```python
from build123d import *

# Parameters (mm, degrees)
F0_W         = 2.23
F0_H         = 8.65
F1_DEPTH     = 1.5
F2_DEPTH     = 31
F5_DEPTH     = 2
F6_R         = 1.5
F7_DEPTH     = 6
F8_R         = 2
F9_DEPTH     = 2.5
F10_T1_DEPTH = 13.5
F10_T3_DEPTH = 36
F10_T6_ANGLE = 90


# Not quite as in the source:
# - a fillet or chamfer that OpenCascade refuses, or shapes differently, is made with other operations: its cross-section is extruded or revolved along the edge and cut away or added
# - a feature names something its author has since deleted; it is built from what else it names


with BuildPart() as f1:
    # F0 (on Top) → F1 (new body)
    with BuildSketch(Plane.XY):
        with BuildLine():
            Line((-1.75, -15), (1.75, -15))
            ThreePointArc((1.75, -15), (3.517766953, -14.267766953), (4.25, -12.5))
            Line((4.25, -12.5), (4.25, -5.3126580607))
            add(Edge.make_bspline(
                [(4.25, -5.3126580607), (5.242489647, 0), (4.25, 5.3126580607)],
                knots=[4.2622339472, 4.2622339472, 4.2622339472, 5.1625440136, 5.1625440136, 5.1625440136], degree=2, weights=[1, 0.9003796574, 1]))
            Line((4.25, 5.3126580607), (4.25, 12.5))
            ThreePointArc((4.25, 12.5), (3.517766953, 14.267766953), (1.75, 15))
            Line((1.75, 15), (-1.75, 15))
            ThreePointArc((-1.75, 15), (-3.517766953, 14.267766953), (-4.25, 12.5))
            Line((-4.25, 12.5), (-4.25, -12.5))
            ThreePointArc((-4.25, -12.5), (-3.517766953, -14.267766953), (-1.75, -15))
        make_face()
        Rectangle(F0_W, F0_H, mode=Mode.SUBTRACT)
    extrude(amount=F1_DEPTH)

    # F0 (on Top) → F2 (join)
    with BuildSketch(Plane.XY):
        with BuildLine():
            ThreePointArc((5.75, 14), (5.017766953, 15.767766953), (3.25, 16.5))
            Line((3.25, 16.5), (-3.25, 16.5))
            ThreePointArc((-3.25, 16.5), (-5.017766953, 15.767766953), (-5.75, 14))
            Line((-5.75, 14), (-5.75, -14))
            ThreePointArc((-5.75, -14), (-5.017766953, -15.767766953), (-3.25, -16.5))
            Line((-3.25, -16.5), (5.75, -16.5))
            Line((5.75, -16.5), (5.75, 14))
        make_face()
        with BuildLine():
            ThreePointArc((4.25, -12.5), (3.517766953, -14.267766953), (1.75, -15))
            Line((1.75, -15), (-1.75, -15))
            ThreePointArc((-1.75, -15), (-3.517766953, -14.267766953), (-4.25, -12.5))
            Line((-4.25, -12.5), (-4.25, 12.5))
            ThreePointArc((-4.25, 12.5), (-3.517766953, 14.267766953), (-1.75, 15))
            Line((-1.75, 15), (1.75, 15))
            ThreePointArc((1.75, 15), (3.517766953, 14.267766953), (4.25, 12.5))
            Line((4.25, 12.5), (4.25, 5.3126580607))
            add(Edge.make_bspline(
                [(4.25, -5.3126580607), (5.242489647, 0), (4.25, 5.3126580607)],
                knots=[4.2622339472, 4.2622339472, 4.2622339472, 5.1625440136, 5.1625440136, 5.1625440136], degree=2, weights=[1, 0.9003796574, 1]))
            Line((4.25, -5.3126580607), (4.25, -12.5))
        make_face(mode=Mode.SUBTRACT)
    extrude(amount=F2_DEPTH)

    # F4 (on face) → F5 (cut)
    with BuildSketch(Plane.YZ.offset(5.75)):
        with BuildLine():
            ThreePointArc((6.52, 16.25), (-4.6103362133, 20.8603362133), (0, 9.73))
            ThreePointArc((0, 9.73), (4.6103362133, 11.6396637867), (6.52, 16.25))
        make_face()
    extrude(amount=-F5_DEPTH, mode=Mode.SUBTRACT)

    # F6
    f6_edges = [f1.edges().sort_by_distance(p)[0] for p in [
        (5.75, -1.25, 0),
    ]]
    fillet(f6_edges, radius=F6_R)

    # F3 (on face) → F7 (join)
    with BuildSketch(Plane.XY.offset(31)):
        with BuildLine():
            Line((2.6164813973, -14.8450394427), (2.6164813973, -16.5))
            Line((2.6164813973, -16.5), (5.75, -16.5))
            Line((5.75, -16.5), (5.75, -13.5683528888))
            Line((5.75, -13.5683528888), (4.0102261181, -13.5683528888))
            ThreePointArc((4.0102261181, -13.5683528888), (3.4386554151, -14.3434866121), (2.6164813973, -14.8450394427))
        make_face()
        with BuildLine():
            Line((4.0102261181, -13.5683528888), (5.75, -13.5683528888))
            Line((5.75, -13.5683528888), (5.75, -9.473525919))
            Line((5.75, -9.473525919), (4.25, -9.473525919))
            Line((4.25, -9.473525919), (4.25, -12.5))
            ThreePointArc((4.25, -12.5), (4.18932012, -13.0474644759), (4.0102261181, -13.5683528888))
        make_face()
        with BuildLine():
            Line((-1.75, -15), (-1.75, -16.5))
            Line((-1.75, -16.5), (2.6164813973, -16.5))
            Line((2.6164813973, -16.5), (2.6164813973, -14.8450394427))
            ThreePointArc((2.6164813973, -14.8450394427), (2.190114413, -14.9609549576), (1.75, -15))
            Line((1.75, -15), (-1.75, -15))
        make_face()
    extrude(amount=F7_DEPTH)

    # F8
    f8_edges = [f1.edges().sort_by_distance(p)[0] for p in [
        (-1.75, -15.75, 37),
        (5, -9.473526, 37),
    ]]
    fillet(f8_edges, radius=F8_R)

    # F3 (on face) → F9 (cut)
    with BuildSketch(Plane.XY.offset(31)):
        with BuildLine():
            Line((2.6164813973, -14.8450394427), (2.6164813973, -16.5))
            Line((2.6164813973, -16.5), (5.75, -16.5))
            Line((5.75, -16.5), (5.75, -13.5683528888))
            Line((5.75, -13.5683528888), (4.0102261181, -13.5683528888))
            ThreePointArc((4.0102261181, -13.5683528888), (3.4386554151, -14.3434866121), (2.6164813973, -14.8450394427))
        make_face()
    extrude(amount=F9_DEPTH, mode=Mode.SUBTRACT)

    # F10: fillet of radius 2 on 2 edges, made by hand

    # F10_s2 → F10_t1 (cut)
    with BuildSketch(Plane.XY.offset(28.5)):
        with BuildLine():
            ThreePointArc((5.75, -14.5), (5.1642135624, -15.9142135624), (3.75, -16.5))
            Line((3.75, -16.5), (5.75, -16.5))
            Line((5.75, -16.5), (5.75, -14.5))
        make_face()
    extrude(amount=F10_T1_DEPTH, mode=Mode.SUBTRACT)

    # F10_s4 → F10_t3 (cut)
    with BuildSketch(Plane.XY):
        with BuildLine():
            ThreePointArc((5.75, -14.5), (5.1642135624, -15.9142135624), (3.75, -16.5))
            Line((3.75, -16.5), (5.75, -16.5))
            Line((5.75, -16.5), (5.75, -14.5))
        make_face()
    extrude(amount=F10_T3_DEPTH, mode=Mode.SUBTRACT)

    # F10_s5 → F10_t6 (revolve, cut)
    with BuildSketch(Plane.XZ.offset(14.5)):
        with BuildLine():
            ThreePointArc((4.25, 0), (5.3106601718, 0.4393398282), (5.75, 1.5))
            Line((5.75, 1.5), (5.75, 0))
            Line((5.75, 0), (4.25, 0))
        make_face()
    revolve(axis=Axis((3.75, -14.5, 0), (0, 0, -1)), revolution_arc=F10_T6_ANGLE, mode=Mode.SUBTRACT)


solid = f1.part
```
For this review, take the finished solid that the model builds, in its own axes (mm). A direction names the side the tool comes from. Round coordinates to 2 decimals unless told otherwise and drop trailing zeros. Write each loop counter-clockwise with the first axis right and the second up, starting at its lowest first coordinate (ties: lowest second). Pieces come first, ordered by that corner, then holes. Notation, with made-up numbers: (68, 41) - (77, 41) arc R13 cw to (77, 63) - close; hole circle Ø10 at (69, -23.75). An arc over 180 degrees is marked (long way). Put each result on its own line as item: value.
Q1. Insertion check: pin 1 Ø0.8 at (y, z) = (0.5, 1) entering from -X; pin 2 Ø4 at (x, y) = (2, -7) entering from +Z; pin 3 Ø0.8 at (y, z) = (-15.5, 33) entering from +X. Each pin has a flat end and moves straight along its axis. Give the tip position at first contact, or say it passes through.
Solved:
pin 1: stops at x = -5.75
pin 2: stops at z = 1.5
pin 3: stops at x = 2.62
Q2. We need section C-C (z = 17.5). Give the boundary of the cut face in (x, y).
Solved:
outline: (-5.75, -14) arc R2.5 ccw to (-3.25, -16.5) - (3.75, -16.5) arc R2 ccw to (5.75, -14.5) - (5.75, -6.4) - (4.25, -6.4) - (4.25, -12.5) arc R2.5 cw to (1.75, -15) - (-1.75, -15) arc R2.5 cw to (-4.25, -12.5) - (-4.25, 12.5) arc R2.5 cw to (-1.75, 15) - (1.75, 15) arc R2.5 cw to (4.25, 12.5) - (4.25, 6.4) - (5.75, 6.4) - (5.75, 14) arc R2.5 ccw to (3.25, 16.5) - (-3.25, 16.5) arc R2.5 ccw to (-5.75, 14) - close
Q3. We need section A-A (z = 32). Give the boundary of the cut face in (x, y).
Solved:
outline: (-1.75, -16.5) - (2.62, -16.5) - (2.62, -14.85) arc R2.5 cw to (1.75, -15) - (-1.75, -15) - close; (4.01, -13.57) - (5.75, -13.57) - (5.75, -9.47) - (4.25, -9.47) - (4.25, -12.5) arc R2.5 cw to start
Q4. Machinability: for faces 1 (the face through (4.25, 9, 16)), 2 (the face through (5, -9.474, 33)), 3 (the face through (-1.75, -16, 33)), 4 (the face through (5, -13.568, 32)), 5 (the face through (0, 4.325, 1)), which of the approach directions +Z, -Z, +X, -X, +Y, -Y give a long, thin tool a straight path to every point of the face, cutting with its end or side? Answer none if there is none.
Solved:
face 1: +Z
face 2: +Z, +X, -X, +Y
face 3: +Z, -X, +Y, -Y
face 4: +X, -X, -Y
face 5: +Z, -Z
Q5. We need section B-B (y = 12). Give the boundary of the cut face in (x, z), and give its area (3 significant figures).
Solved:
outline: (-5.75, 1.5) arc R1.5 ccw to (-4.25, 0) - (4.25, 0) arc R1.5 ccw to (5.75, 1.5) - (5.75, 31) - (4.25, 31) - (4.25, 1.5) - (-4.25, 1.5) - (-4.25, 31) - (-5.75, 31) - close
area: 105 mm2
Q6. We need section D-D (y = -13). Give the boundary of the cut face in (x, z), and give its area (3 significant figures).
Solved:
outline: (-5.75, 1.5) arc R1.5 ccw to (-4.25, 0) - (4.25, 0) arc R1.5 ccw to (5.75, 1.5) - (5.75, 37) - (4.2, 37) - (4.2, 1.5) - (-4.2, 1.5) - (-4.2, 31) - (-5.75, 31) - close
area: 117 mm2
Q7. Mouldability with a two-part tool opening along Y and no side actions: class faces 6 (the face through (4.25, -9, 19)), 7 (the face through (5.18, -15.9, 16.04)), 8 (the face through (-5.75, 0, 16)) as released by +Y, released by -Y, zero draft, split by the parting line, or undercut.
Solved:
face 6: undercut
face 7: released by -Y
face 8: zero draft
Q8. Wall thickness on probe 1 along X at (y, z) = (-10, 3); probe 2 along Y at (x, z) = (1.5, 23): over which ranges is each line inside the solid? List them lowest first.
Solved:
probe 1: x = -5.75 to -4.25, 4.25 to 5.75
probe 2: y = -16.5 to -15, 15 to 16.5
